```python
from build123d import *

# Parameters (mm, degrees)
EXTRUDE_1_DEPTH = 920
FILLET_1_R      = 10
SHELL_1_T       = -2


with BuildPart() as part:
    # 草图1 → 凸台-拉伸1 (new body)
    with BuildSketch(Plane.XY):
        with BuildLine():
            Line((-175, 0), (175, 0))
            ThreePointArc((175, 0), (0, 175), (-175, 0))
        make_face()
    extrude(amount=EXTRUDE_1_DEPTH)

    # 圆角1
    fillet_1_edges = [part.edges().sort_by_distance(p)[0] for p in [
        (0, 175, 920),
    ]]
    fillet(fillet_1_edges, radius=FILLET_1_R)

    # 抽壳1
    shell_1_openings = [part.faces().sort_by_distance(p)[0] for p in [
        (0, 0, 459.938974789),
    ]]
    offset(amount=SHELL_1_T, openings=shell_1_openings)


solid = part.part
```
Could you check a few things on this model? Use its own coordinates, in mm. A direction names the side the tool comes from. Round coordinates to 2 decimals unless told otherwise and drop trailing zeros. Loops run counter-clockwise (first coordinate to the right, second up) from the corner with the lowest first, then second, coordinate; pieces in that order, holes last. Notation, with made-up numbers: (26.5, 28.5) -> (68.5, 28.5) arc R18 cw to (68.5, 63.5) -> close; hole circle Ø8 at (-14, -16). An arc over 180 degrees is marked (long way). Put each result on its own line as item: value.
Q1. Which directions (+Z, -Z, +X, -X, +Y, -Y) give clear straight access to the entire face, cutting with the end or side of a thin tool? Please do faces 4 (the cylindrical face through (3.8, 172.96, 449.64)), 5 (the flat face through (-2, 65, 920)).
Checks:
face 4: -Y
face 5: +Z, +X, -X, +Y, -Y
Q2. For pin 1 Ø12 at (y, z) = (52, 756) entering from -X; pin 2 Ø5 at (y, z) = (61, 724) entering from -X; pin 3 Ø12 at (y, z) = (118, 488.5) entering from +X, each with a flat end and sliding along its axis, tell me the tip position at first contact or that it passes through.
Checks:
pin 1: x = -168.85
pin 2: x = -164.93
pin 3: x = 134.47
Q3. Thinking about a two-plate mould opening in X: for faces 1 (the cylindrical face through (3.848, 174.958, 448.63)), 2 (the flat face through (-2, 69, 0)), 3 (the flat face through (-2, 68, 2)), which applies, pulls with the +X half, pulls with the -X half, needs draft (parallel to the pull), parting line crosses it, or undercut?
Checks:
face 1: parting line crosses it
face 2: needs draft
face 3: undercut
Q4. I want a section at A-A on z = 67. Write out the boundary of the cut face in (x, y), and give its area (3 significant figures).
Checks:
outline: (-175, 0) -> (-173, 0) arc R173 cw to (173, 0) -> (175, 0) arc R175 ccw to start
area: 1,090 mm2
Q5. Please list where these lines run through material, in increasing order: line 1 (Z direction, x = 20, y = 131.5); line 2 (Z direction, x = -113, y = 129); line 3 (X direction, y = 38, z = 187.5) (3 decimals). Write a range as from..to.
Checks:
line 1: 0..2, 918..920
line 2: 0..2, 914.67..917.6
line 3: -170.824..-168.775, 168.775..170.824
